Input: part model. Units: mm. Frame: model coordinates. Face numbers are marked on the shaded views. Round coordinates to 2 decimals unless told otherwise and drop trailing zeros. Order: outer loops, then holes, each group sorted by start corner. A loop starts at its lowest first (then second) coordinate and runs counter-clockwise, first axis right, second up.
Item 1: Cut plane B-B on y = -30. Output: boundary loops of the cut face in (x, z), then the cut area to 3 significant figures.
Item 2: Cut plane D-D on y = 1.44. Output: boundary loops of the cut face in (x, z) (3 decimals), then the cut area to 3 significant figures.
Item 3: Mould query, pull axis Y, two halves, no side actions, for the marked faces 1 and 2. Classes: released by +Y, released by -Y, zero draft, split by the parting line, or undercut.
Item 4: First-contact query: pin 1 (6 mm diameter, centred on x = -30.5, y = 34, fed in from +Z); pin 2 (1.4 mm diameter, centred on y = 66, z = -1, fed in from +X); pin 3 (0.6 mm diameter, centred on y = -66, z = -1.5, fed in from -X); pin 4 (0.6 mm diameter, centred on x = -50, z = -2, fed in from +Y). Flat tips, straight axial feed; report the tip coordinate or a pass-through.
Item 5: Line query: L1, parallel to X at y = -57.5, z = -0.5; L2, parallel to Z at x = -22.5, y = -33.5. Output: solid intervals per line, ascending.
Item 6: Cut plane C-C on z = 16. Output: boundary loops of the cut face in (x, y) (3 decimals), then the cut area to 3 significant figures.
Item 7: Cut plane A-A on x = 3. Output: boundary loops of the cut face in (y, z).
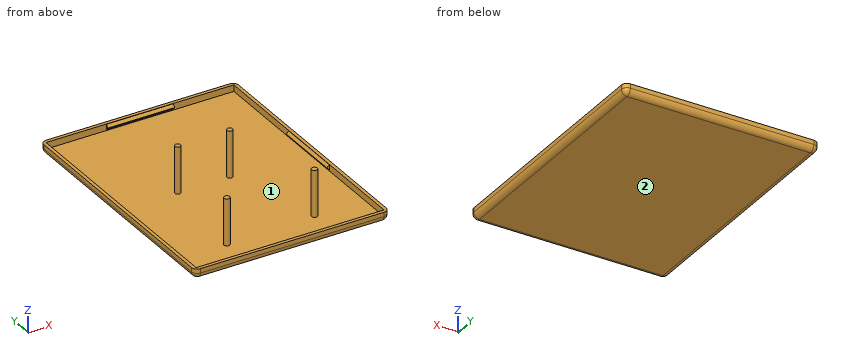
```python
from build123d import *

# Parameters (mm, degrees)
ESQUISSE1_W        = 101.2
ESQUISSE1_H        = 133.2
BOSS_EXTRU_1_DEPTH = 3.5
COQUE1_T           = 1.8
CONG_4_R           = 3
BOSS_EXTRU_2_DEPTH = 18
BOSS_EXTRU_3_DEPTH = 18
ESQUISSE5_R        = 1.55
BOSS_EXTRU_4_DEPTH = 25


with BuildPart() as part:
    # Esquisse1 → Boss.-Extru.1 (new body)
    with BuildSketch(Plane.XY):
        Rectangle(ESQUISSE1_W, ESQUISSE1_H)
    extrude(amount=-BOSS_EXTRU_1_DEPTH)

    # Coque1
    coque1_openings = [part.faces().sort_by_distance(p)[0] for p in [
        (0, 0, 0),
    ]]
    offset(amount=COQUE1_T, openings=coque1_openings, kind=Kind.INTERSECTION)

    # Congé4
    # the kernel refuses this fillet: 3 mm, written as the material it takes off along each edge
    with BuildSketch(Plane(origin=(-49.4, -65.4, -2.3), x_dir=(0, 0, -1), z_dir=(-1, 0, 0))) as cong_4_piece_1_section:
        Polygon((0, 0), (CONG_4_R, 0), (CONG_4_R, CONG_4_R), (0, CONG_4_R), align=None)
    cong_4_piece_1 = extrude(amount=CONG_4_R, mode=Mode.PRIVATE)
    cong_4_piece_1 = cong_4_piece_1 - Plane(origin=(-49.4, -65.4, -2.3), x_dir=(0, 0.7071067811865475, 0.7071067811865475), z_dir=(-1, 0, 0)) * Sphere(CONG_4_R, mode=Mode.PRIVATE)
    add(cong_4_piece_1, mode=Mode.SUBTRACT)
    with BuildSketch(Plane(origin=(-49.4, 65.4, -2.3), x_dir=(-1, 0, 0), z_dir=(0, 1, 0))) as cong_4_piece_2_section:
        Polygon((0, 0), (CONG_4_R, 0), (CONG_4_R, -CONG_4_R), (0, -CONG_4_R), align=None)
    cong_4_piece_2 = extrude(amount=CONG_4_R, mode=Mode.PRIVATE)
    cong_4_piece_2 = cong_4_piece_2 - Plane(origin=(-49.4, 65.4, -2.3), x_dir=(0.7071067811865475, 0, 0.7071067811865475), z_dir=(0, 1, 0)) * Sphere(CONG_4_R, mode=Mode.PRIVATE)
    add(cong_4_piece_2, mode=Mode.SUBTRACT)
    with BuildSketch(Plane(origin=(49.4, -65.4, -2.3), x_dir=(0, -1, 0), z_dir=(0, 0, -1))) as cong_4_piece_3_section:
        Polygon((0, 0), (CONG_4_R, 0), (CONG_4_R, -CONG_4_R), (0, -CONG_4_R), align=None)
    cong_4_piece_3 = extrude(amount=CONG_4_R, mode=Mode.PRIVATE)
    cong_4_piece_3 = cong_4_piece_3 - Plane(origin=(49.4, -65.4, -2.3), x_dir=(-0.7071067811865475, 0.7071067811865475, 0), z_dir=(0, 0, -1)) * Sphere(CONG_4_R, mode=Mode.PRIVATE)
    add(cong_4_piece_3, mode=Mode.SUBTRACT)
    with BuildSketch(Plane(origin=(49.4, 65.4, -2.3), x_dir=(0, 0, -1), z_dir=(0, 1, 0))) as cong_4_piece_4_section:
        Polygon((0, 0), (CONG_4_R, 0), (CONG_4_R, -CONG_4_R), (0, -CONG_4_R), align=None)
    cong_4_piece_4 = extrude(amount=CONG_4_R, mode=Mode.PRIVATE)
    cong_4_piece_4 = cong_4_piece_4 - Plane(origin=(49.4, 65.4, -2.3), x_dir=(-0.7071067811865475, 0, 0.7071067811865475), z_dir=(0, 1, 0)) * Sphere(CONG_4_R, mode=Mode.PRIVATE)
    add(cong_4_piece_4, mode=Mode.SUBTRACT)
    with BuildSketch(Plane(origin=(-52.4, -65.4, -5.3), x_dir=(0, 0, 1), z_dir=(0, 1, 0)), Plane(origin=(52.4, 65.4, -5.3), x_dir=(0, 0, 1), z_dir=(0, -1, 0))) as cong_4_piece_5:
        with BuildLine():
            CenterArc((CONG_4_R, CONG_4_R), CONG_4_R, 180, 90)
            Line((0, CONG_4_R), (0, 0))
            Line((0, 0), (CONG_4_R, 0))
        make_face()
    extrude(amount=130.8, mode=Mode.SUBTRACT)
    with BuildSketch(Plane(origin=(49.4, -68.4, -5.3), x_dir=(0, 0, 1), z_dir=(-1, 0, 0)), Plane(origin=(-49.4, 68.4, -5.3), x_dir=(0, 0, 1), z_dir=(1, 0, 0))) as cong_4_piece_6:
        with BuildLine():
            CenterArc((CONG_4_R, CONG_4_R), CONG_4_R, 180, 90)
            Line((0, CONG_4_R), (0, 0))
            Line((0, 0), (CONG_4_R, 0))
        make_face()
    extrude(amount=98.8, mode=Mode.SUBTRACT)
    with BuildSketch(Plane(origin=(52.4, -68.4, -2.3), x_dir=(-1, 0, 0), z_dir=(0, 0, 1)), Plane(origin=(-52.4, -68.4, 7.5), x_dir=(1, 0, 0), z_dir=(0, 0, -1)), Plane(origin=(-52.4, 68.4, -2.3), x_dir=(1, 0, 0), z_dir=(0, 0, 1)), Plane(origin=(52.4, 68.4, -2.3), x_dir=(0, -1, 0), z_dir=(0, 0, 1))) as cong_4_piece_7:
        with BuildLine():
            CenterArc((CONG_4_R, -CONG_4_R), CONG_4_R, 90, 90)
            Line((0, -CONG_4_R), (0, 0))
            Line((0, 0), (CONG_4_R, 0))
        make_face()
    extrude(amount=9.8, mode=Mode.SUBTRACT)

    # Esquisse3D1 → Boss.-Extru.2 (add, symmetric)
    with BuildSketch(Plane(origin=(50.6, 0, -0.15), x_dir=(0, 0, -1), z_dir=(0, 1, 0))):
        Polygon((0, 0), (2.8, 0), (1.4, 1.284523258), align=None)
    boss_extru_2 = extrude(amount=BOSS_EXTRU_2_DEPTH, both=True)

    # Symétrie1: Boss.-Extru.2 across plane
    add(boss_extru_2.mirror(Plane(origin=(0, 0, 0), x_dir=(0, 0, 1), z_dir=(1, 0, 0))))

    # Esquisse3D2 → Boss.-Extru.3 (add, symmetric)
    with BuildSketch(Plane(origin=(0, 66.6, -0.15), x_dir=(0, 0, -1), z_dir=(-1, 0, 0))):
        Polygon((0, 0), (2.8, 0), (1.4, 1.284523258), align=None)
    boss_extru_3 = extrude(amount=BOSS_EXTRU_3_DEPTH, both=True)

    # Symétrie2: Boss.-Extru.3 across plane
    add(boss_extru_3.mirror(Plane.ZX))

    # Esquisse5 → Boss.-Extru.4 (add)
    with BuildSketch(Plane.XY.offset(-3.5)):
        with Locations(Location((-24.345, -50.63, 0), (0, 0, 180))):
            Circle(ESQUISSE5_R)
        with Locations(Location((23.585, -49.36, 0), (0, 0, 180))):
            Circle(ESQUISSE5_R)
        with Locations(Location((8.835, 1.44, 0), (0, 0, 180))):
            Circle(ESQUISSE5_R)
        with Locations(Location((-19.205, 1.44, 0), (0, 0, 180))):
            Circle(ESQUISSE5_R)
    extrude(amount=BOSS_EXTRU_4_DEPTH)


solid = part.part
```
From the geometry:
1. outline: (-52.4, -2.3) arc R3 ccw to (-49.4, -5.3) - (49.4, -5.3) arc R3 ccw to (52.4, -2.3) - (52.4, 0) - (50.6, 0) - (50.6, -3.5) - (-50.6, -3.5) - (-50.6, 0) - (-52.4, 0) - close
1. area: 197 mm2
2. outline: (-52.4, -2.3) arc R3 ccw to (-49.4, -5.3) - (49.4, -5.3) arc R3 ccw to (52.4, -2.3) - (52.4, 0) - (50.6, 0) - (50.6, -0.15) - (49.315, -1.55) - (50.6, -2.95) - (50.6, -3.5) - (10.385, -3.5) - (10.385, 21.5) - (7.285, 21.5) - (7.285, -3.5) - (-17.655, -3.5) - (-17.655, 21.5) - (-20.755, 21.5) - (-20.755, -3.5) - (-50.6, -3.5) - (-50.6, -2.95) - (-49.315, -1.55) - (-50.6, -0.15) - (-50.6, 0) - (-52.4, 0) - close
2. area: 356 mm2
3. face 1: undercut
3. face 2: zero draft
4. pin 1: stops at z = -3.5
4. pin 2: stops at x = 52.4
4. pin 3: stops at x = -52.38
4. pin 4: stops at y = 68.38
5. L1: x = -52.4 to -50.6, 50.6 to 52.4
5. L2: z = -5.3 to -3.5
6. outline: circle Ø3.1 at (-24.345, -50.63); circle Ø3.1 at (-19.205, 1.44); circle Ø3.1 at (8.835, 1.44); circle Ø3.1 at (23.585, -49.36)
6. area: 30.2 mm2
7. outline: (-68.4, -2.3) arc R3 ccw to (-65.4, -5.3) - (65.4, -5.3) arc R3 ccw to (68.4, -2.3) - (68.4, 0) - (66.6, 0) - (66.6, -0.15) - (65.32, -1.55) - (66.6, -2.95) - (66.6, -3.5) - (-66.6, -3.5) - (-66.6, -2.95) - (-65.32, -1.55) - (-66.6, -0.15) - (-66.6, 0) - (-68.4, 0) - close
